Autodesk Inventor part; units mm, degrees
ref_plane "YZ Plane" through (0, 0, 0) normal (1, 0, 0) x (0, 1, 0)
ref_plane "XZ Plane" through (0, 0, 0) normal (0, 1, 0) x (-1, 0, 0)
ref_plane "XY Plane" through (0, 0, 0) normal (0, 0, 1) x (1, 0, 0)
sketch "Sketch2" plane through (0, 0, 0) normal (0, 0, 1) x (1, 0, 0)
  line L0 (-17, 28) -> (0, 28)
  line L1 (0, 28) -> (0, 17)
  line L2 (0, 7) -> (0, 0)
  line L3 (0, 0) -> (-17, 0)
  line L4 (-17, 0) -> (-17, 7)
  line L5 (-17, 28) -> (-17, 17)
  line L6 (-17, 17) -> (-17, 7)
  line L7 (0, 17) -> (0, 7)
  dimension "d0" = 17
  dimension "d1" = 28
extrude "Extrusion1" add sketch "Sketch2" along normal blind 5
sketch "Sketch4" plane through (0, 0, 0) normal (0, 0, -1) x (-1, 0, 0)
  line L0 (17, 28) -> (0, 28)
  line L1 (0, 28) -> (0, 0)
  line L2 (0, 0) -> (17, 0)
  line L3 (17, 0) -> (17, 28)
  line L4 (0, 28) -> (17, 28)
  line L5 (11.5, 24) -> (11.5, 4)
  line L6 (11.5, 4) -> (5.5, 4)
  line L7 (5.5, 4) -> (5.5, 24)
  line L8 (5.5, 24) -> (11.5, 24)
  dimension "d15" = 6
  dimension "d17" = 5.5
  dimension "d30" = 20
  dimension "d31" = 4
extrude "Extrusion3" cut sketch "Sketch4" against normal blind 1.5 contours L5 L6 L7 L8
sketch "Sketch5" plane through (0, 0, 5) normal (0, 0, 1) x (1, 0, 0)
  line L0 (0, 28) -> (-17, 28)
  line L1 (-17, 28) -> (-17, 0)
  line L2 (-17, 0) -> (0, 0)
  line L3 (0, 0) -> (0, 28)
  line L4 (-21, 17) -> (4, 7)
  line L5 (-21.4753, 7) -> (4, 17)
  circle A0 centre (-8.6177, 12.0471) radius 5
  dimension "d20" = 10
  dimension "d21" = 12.0471
extrude "Extrusion4" cut sketch "Sketch5" against normal through all contours A0 L4 L5 | L5 L4 A0 | L4 L5 A0 | A0 L5 L4
sketch "Sketch6" plane through (0, 0, 5) normal (0, 0, 1) x (1, 0, 0)
  circle A0 centre (-8.6177, 12.0471) radius 5
  line L0 (0, 28) -> (-17, 28)
  line L1 (-17, 28) -> (-17, 0)
  line L2 (-17, 0) -> (0, 0)
  line L3 (0, 0) -> (0, 28)
  circle A1 centre (-12.5, 26) radius 1.35
  dimension "d24" = 2.7
  dimension "d25" = 4.5
  dimension "d26" = 2
extrude "Extrusion5" cut sketch "Sketch6" against normal through all contours A1
sketch "Sketch7" plane through (0, 0, 5) normal (0, 0, 1) x (1, 0, 0)
  line L0 (0, 0) -> (0, 28)
  line L1 (-17, 0) -> (0, 0)
  circle A0 centre (-4.5, 5) radius 1.35
  point P0 (0, 7)
  dimension "d32" = 2.7
  dimension "d33" = 4.5
  dimension "d34" = 5
extrude "Extrusion6" cut sketch "Sketch7" against normal through all
sketch "Sketch8" plane through (0, 0, 0) normal (1, 0, 0) x (0, 0, -1)
  circle A0 centre (-2.5, 11.5) radius 1.6
  line L0 (-5, 0) -> (-5, 28)
  line L1 (0, 0) -> (-5, 0)
  point P0 (0, -7)
  dimension "d37" = 3.2
  dimension "d41" = 11.5
  dimension "d49" = 2.5
extrude "Extrusion8" cut sketch "Sketch8" against normal through all
sketch "Sketch9" plane through (0, 0, 5) normal (0, 0, 1) x (1, 0, 0)
  circle A0 centre (-4.5, 5) radius 1.35
  circle A1 centre (-12.5, 26) radius 1.35
  circle A2 centre (-8.6177, 12.0471) radius 5
  line L0 (0, 28) -> (-17, 28)
  line L1 (-17, 28) -> (-17, 0)
  line L2 (-17, 0) -> (0, 0)
  line L3 (0, 0) -> (0, 28)
  line L4 (-17, 0) -> (-16.5, 0)
  line L5 (-16.5, 0) -> (-16.5, 28)
  line L6 (-16.5, 28) -> (-17, 28)
  line L7 (-17, 28) -> (-17, 0)
  line L8 (0, 0) -> (-0.5, 0)
  line L9 (-0.5, 0) -> (-0.5, 28)
  line L10 (-0.5, 28) -> (0, 28)
  line L11 (0, 28) -> (0, 0)
  dimension "d47" = 0.5
  dimension "d48" = 0.5
extrude "Extrusion9" cut sketch "Sketch9" against normal through all contours L3 L2 L9 L0 | L5 L2 L1 L0
properties part number "tapaA0.2"
Build history of the part. All positions in model axes, mm. A direction names the side the tool comes from. Round coordinates to 2 decimals unless told otherwise and drop trailing zeros. Write each loop counter-clockwise with the first axis right and the second up, starting at its lowest first coordinate (ties: lowest second). Pieces come first, ordered by that corner, then holes.
1) 3-axis set-ups, long thin cutter, end or side, ignore diameter. For faces 5 (the cylindrical face through (-12.79, 24.68, 2.54)), 6 (the flat face through (-11.5, 6, 1)): which of +Z, -Z, +X, -X, +Y, -Y reach the whole face in a straight line?
2) Pin check, flat tip, straight feed: pin 1 (2 mm diameter, centred on x = -8, y = 5.5, fed in from -Z). Stop position of the tip, or through.
3) Band-saw the part on D-D, the plane y = 10.25. List the corners of the cut face in (x, z).
4) Mould opens along X. For faces 1 (the flat face through (-9, 28, 2)), 2 (the flat face through (-11.5, 20, 1)), 3 (the flat face through (-0.5, 14, 3)), 4 (the flat face through (-8, 20, 1.5)) say: +X half, -X half, draft (parallel to the pull), parting line (faces both ways), or undercut.
5) Drill centre lines: probe 1 along Y at (x, z) = (-8, 0.3); probe 2 along Y at (x, z) = (-3, 2.4); probe 3 along Y at (x, z) = (-4.5, 0.5). Where is each one in solid material? Low to high.
6) Band-saw the part on C-C, the plane x = -4.5. List the corners of the cut face in (y, z).
7) Band-saw the part on A-A, the plane y = 26. List the corners of the cut face in (x, z), and give its area (3 significant figures).
8) Band-saw the part on B-B, the plane z = 3.1. List the corners of the cut face in (x, y), and give its area (3 significant figures).
Ans:
1. face 5: +Z, -Z
1. face 6: -Z
2. pin 1: stops at z = 1.5
3. outline: (-16.5, 0) - (-13.28, 0) - (-13.28, 1.5) - (-16.5, 1.5) - close; (-16.5, 3.5) - (-13.28, 3.5) - (-13.28, 5) - (-16.5, 5) - close; (-3.95, 0) - (-0.5, 0) - (-0.5, 1.5) - (-3.95, 1.5) - close; (-3.95, 3.5) - (-0.5, 3.5) - (-0.5, 5) - (-3.95, 5) - close
4. face 1: draft
4. face 2: undercut
4. face 3: +X half
4. face 4: undercut
5. probe 1: y = 0 to 4, 24 to 28
5. probe 2: y = 0 to 9.9, 13.1 to 28
5. probe 3: y = 0 to 3.65, 6.35 to 9.21, 14.88 to 28
6. outline: (0, 0) - (3.65, 0) - (3.65, 5) - (0, 5) - close; (6.35, 0) - (9.21, 0) - (9.21, 5) - (6.35, 5) - close; (14.88, 0) - (28, 0) - (28, 5) - (14.88, 5) - close
7. outline: (-16.5, 0) - (-13.85, 0) - (-13.85, 5) - (-16.5, 5) - close; (-11.15, 0) - (-0.5, 0) - (-0.5, 5) - (-11.15, 5) - close
7. area: 66.5 mm2
8. outline: (-16.5, 0) - (-0.5, 0) - (-0.5, 10.02) - (-4.05, 10.02) arc R5 cw to (-13.19, 10.02) - (-16.5, 10.02) - close; (-16.5, 12.98) - (-13.53, 12.98) arc R5 cw to (-3.71, 12.98) - (-0.5, 12.98) - (-0.5, 28) - (-16.5, 28) - close; hole circle Ø2.7 at (-12.5, 26); hole circle Ø2.7 at (-4.5, 5)
8. area: 340 mm2
